Geometry: final body of the model. Coordinates: model frame, mm. A direction names the side the tool comes from. Coordinates: 2 decimals unless noted, no trailing zeros. Write each loop counter-clockwise with the first axis right and the second up, starting at its lowest first coordinate (ties: lowest second). Pieces come first, ordered by that corner, then holes. Notation, with made-up numbers: (-20.5, 43) - (-1.5, 43) arc R15 cw to (-1.5, 49) - close; hole circle Ø6 at (77.5, -28). An arc over 180 degrees is marked (long way). Put each result on its own line as item: value.
```python
from build123d import *

# Parameters (mm, degrees)
SKETCH1_R           = 3.55
BOSS_EXTRUDE1_DEPTH = 1
SKETCH3_R           = 3.1
BOSS_EXTRUDE2_DEPTH = 15


with BuildPart() as part:
    # Sketch1 → Boss-Extrude1 (new body)
    with BuildSketch(Plane(origin=(0, 0, 0), x_dir=(1, 0, 0), z_dir=(0, 1, 0))):
        with Locations(Location((0, 0, 0), (0, 0, 270))):
            Circle(SKETCH1_R)
    extrude(amount=BOSS_EXTRUDE1_DEPTH)

    # Sketch2 → Revolve1 (revolve)
    with BuildSketch(Plane(origin=(0, 0, 0), x_dir=(0, 0, -1), z_dir=(1, 0, 0))):
        with BuildLine():
            Line((0, 1), (0, 4))
            ThreePointArc((0, 4), (2.121320344, 3.121320344), (3, 1))
            Line((3, 1), (0, 1))
        make_face()
    revolve(axis=Axis((0, 1, 0), (0, -1, 0)))

    # Sketch3 → Boss-Extrude2 (add)
    with BuildSketch(Plane.XZ):
        with Locations(Location((0, 0, 0), (0, 0, 90))):
            Circle(SKETCH3_R)
    extrude(amount=BOSS_EXTRUDE2_DEPTH)


solid = part.part
```
1. Pin query (flat end, axial travel): pin 1 Ø3 at (y, z) = (-7.5, -1.5) entering from -X; pin 2 Ø2 at (x, z) = (0.5, 3) entering from +Y. Return the tip coordinate at first contact, or that it passes through.
Answer below:
pin 1: stops at x = -3.1
pin 2: stops at y = 3.2
2. Section query B-B (z = 0). Return loops of the section in (x, y).
Answer below:
outline: (-3.55, 0) - (-3.1, 0) - (-3.1, -15) - (3.1, -15) - (3.1, 0) - (3.55, 0) - (3.55, 1) - (3, 1) arc R3 ccw to (-3, 1) - (-3.55, 1) - close
3. Section query D-D (z = 2). Return loops of the section in (x, y).
Answer below:
outline: (-2.93, 0) - (-2.37, 0) - (-2.37, -15) - (2.37, -15) - (2.37, 0) - (2.93, 0) - (2.93, 1) - (2.24, 1) arc R2.24 ccw to (-2.24, 1) - (-2.93, 1) - close
4. Section query A-A (x = 0). Return loops of the section in (y, z).
Answer below:
outline: (-15, -3.1) - (0, -3.1) - (0, -3.55) - (1, -3.55) - (1, -3) arc R3 ccw to (1, 3) - (1, 3.55) - (0, 3.55) - (0, 3.1) - (-15, 3.1) - close
5. Section query C-C (y = -4). Return loops of the section in (x, z), then the cut area to 3 significant figures.
Answer below:
outline: circle Ø6.2 at (0, 0)
area: 30.2 mm²
6. Set-up query: faces 1 (the flat face through (3, 1, -1)), 2 (the cylindrical face through (3, 0.5, 1.9)), 3 (the cylindrical face through (-0.931, -7.395, 2.957)). Return all of +Z, -Z, +X, -X, +Y, -Y with unobstructed straight access to the full face (end or side cutting, diameter ignored); none if empty.
Answer below:
face 1: +Y
face 2: +Y, -Y
face 3: -Y
7. Ray query, probe 1 along X at (y, z) = (-2.25, -1.75); probe 2 along Y at (x, z) = (1.5, 0.75); probe 3 along Z at (x, y) = (-1, -4). Return the intervals inside material, ascending. Write a range as from..to.
Answer below:
probe 1: x = -2.56..2.56
probe 2: y = -15..3.49
probe 3: z = -2.93..2.93
